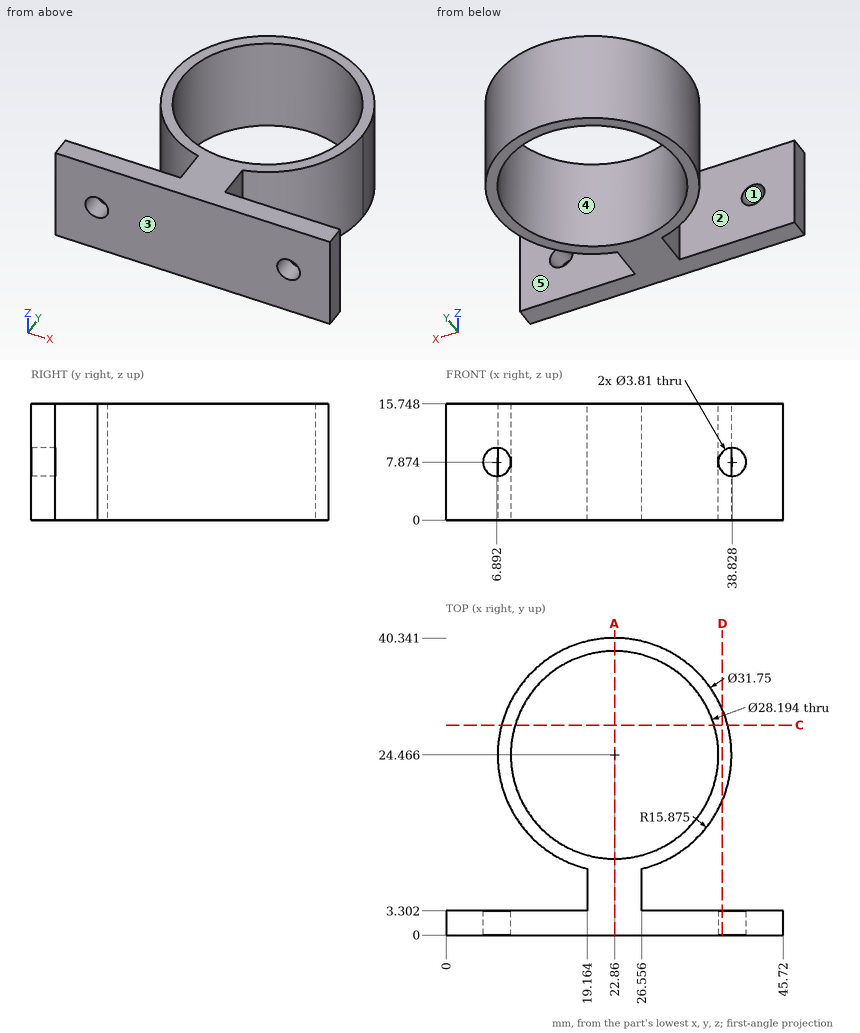
Check sheet for the drawn part. Datum: minimum x, y, z corner. Units: mm. A direction names the side the tool comes from. Coordinates: 2 decimals unless noted, no trailing zeros. Order: outer loops, then holes, each group sorted by start corner. A loop starts at its lowest first (then second) coordinate and runs counter-clockwise, first axis right, second up. Notation, with made-up numbers: (49.25, -7.75) -> (78.25, -7.75) arc R27 cw to (78.25, 14.25) -> close; hole circle Ø3 at (8.25, -9). An arc over 180 degrees is marked (long way). Use a Markdown table: item, result. Add a question column.
1. Cross-section at C-C (y = 28.5). Enter the section's corners in (x, z).
2. Material ranges on L1, parallel to Y at x = 22.86, z = 4; L2, parallel to X at y = 24.5, z = 7.5 (1 decimal); L3, parallel to X at y = 13, z = 1.5, recorded low to high.
3. Go/stop test with flat-tipped pins: pin 1 Ø2.5 at (x, z) = (6.89, 7.87) entering from -Y (1 decimal); pin 2 Ø5 at (x, z) = (29, 9) entering from +Y; pin 3 Ø1.5 at (y, z) = (22, 12) entering from -X. Record where each tip stops, or that it passes through.
4. Set-up check for the marked faces 4 and 5: record each of +Z, -Z, +X, -X, +Y, -Y from which the full face is reachable in a straight line by a thin tool's end or side.
5. Cross-section at D-D (x = 37.5). Enter the section's corners in (y, z) (1 decimal), and give its area (3 significant figures).
6. Cross-section at A-A (x = 22.86). Enter the section's corners in (y, z).
7. Mould release check, pull along Y, two halves, no side actions. Record for the marked faces 1, 2 and 3: pulls with the +Y half, pulls with the -Y half, needs draft (parallel to the pull), parting line crosses it, or undercut.
Filled sheet:
| question | item | result |
|---|---|---|
| 1 | outline | (7.51, 0) -> (9.35, 0) -> (9.35, 15.75) -> (7.51, 15.75) -> close; (36.37, 0) -> (38.21, 0) -> (38.21, 15.75) -> (36.37, 15.75) -> close |
| 2 | L1 | 0 to 10.37, 38.56 to 40.34 |
| 2 | L2 | 7 to 8.8, 37 to 38.7 |
| 2 | L3 | 11.88 to 14.66, 31.06 to 33.84 |
| 3 | pin 1 | y = 18.5 |
| 3 | pin 2 | y = 39.92 |
| 3 | pin 3 | x = 7.08 |
| 4 | face 4 | +Z, -Z |
| 4 | face 5 | +Z, -Z, +X |
| 5 | outline | (0, 0) -> (3.3, 0) -> (3.3, 6.5) -> (0, 6.5) -> close; (0, 9.2) -> (3.3, 9.2) -> (3.3, 15.7) -> (0, 15.7) -> close; (18.3, 0) -> (30.6, 0) -> (30.6, 15.7) -> (18.3, 15.7) -> close |
| 5 | area | 236 mm2 |
| 6 | outline | (0, 0) -> (10.37, 0) -> (10.37, 15.75) -> (0, 15.75) -> close; (38.56, 0) -> (40.34, 0) -> (40.34, 15.75) -> (38.56, 15.75) -> close |
| 7 | face 1 | needs draft |
| 7 | face 2 | undercut |
| 7 | face 3 | pulls with the -Y half |
